Check sheet for the drawn part. Datum: minimum x, y, z corner. Units: mm. Coordinates: 2 decimals unless noted, no trailing zeros. Write each loop counter-clockwise with the first axis right and the second up, starting at its lowest first coordinate (ties: lowest second). Pieces come first, ordered by that corner, then holes. Notation, with made-up numbers: (21.5, 82.5) - (56.5, 82.5) arc R30 ccw to (56.5, 114.5) - close; hole circle Ø1 at (75.25, -38.75). An arc over 180 degrees is marked (long way). Use one line per item in the form item = value. Start each with the question number.
1. Cross-section at C-C on x = 20. Record the boundary of the cut face in (y, z).
2. Cross-section at A-A on x = 38.1. Record the boundary of the cut face in (y, z), then the cut area to 3 significant figures.
3. Scan lines: line 1 along X through (y, z) = (110, 1.85); line 2 along Y through (x, z) = (38.1, 0.8); line 3 along X through (y, z) = (108, 2.85). Record each from-to range of solid material in increasing order.
4. Go/stop test with a flat-tipped pin: pin 1 Ø4.5 at (x, y) = (14.53, 14.605) entering from +Z. Record where the tip stops, or that it passes through.
5. Cross-section at B-B on z = 2.7. Record the boundary of the cut face in (x, y) (3 decimals).
6. Cross-section at D-D on y = 22. Record the boundary of the cut face in (x, z), then the cut area to 3 significant figures.
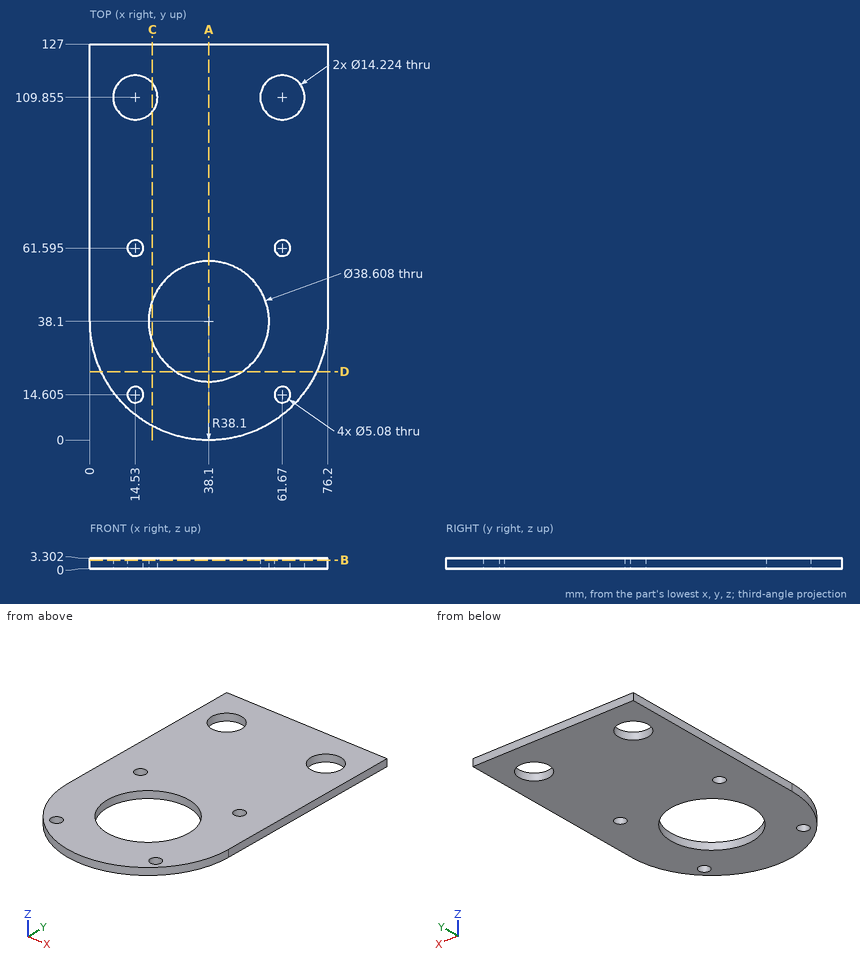
Final values:
q1.outline = (4.57, 0) - (31.39, 0) - (31.39, 3.3) - (4.57, 3.3) - close; (44.81, 0) - (105.31, 0) - (105.31, 3.3) - (44.81, 3.3) - close; (114.4, 0) - (127, 0) - (127, 3.3) - (114.4, 3.3) - close
q2.outline = (0, 0) - (18.8, 0) - (18.8, 3.3) - (0, 3.3) - close; (57.4, 0) - (127, 0) - (127, 3.3) - (57.4, 3.3) - close
q2.area = 292 mm²
q3.line_1 = 0 to 7.42, 21.64 to 54.56, 68.78 to 76.2
q3.line_2 = 0 to 18.8, 57.4 to 127
q3.line_3 = 0 to 7.66, 21.4 to 54.8, 68.54 to 76.2
q4.pin_1 = through
q5.outline = (0, 38.1) arc R38.1 ccw to (76.2, 38.1) - (76.2, 127) - (0, 127) - close; hole circle Ø14.224 at (14.53, 109.855); hole circle Ø5.08 at (14.53, 14.605); hole circle Ø5.08 at (14.53, 61.595); hole circle Ø38.608 at (38.1, 38.1); hole circle Ø14.224 at (61.67, 109.855); hole circle Ø5.08 at (61.67, 14.605); hole circle Ø5.08 at (61.67, 61.595)
q6.outline = (3.57, 0) - (27.45, 0) - (27.45, 3.3) - (3.57, 3.3) - close; (48.75, 0) - (72.63, 0) - (72.63, 3.3) - (48.75, 3.3) - close
q6.area = 158 mm²
